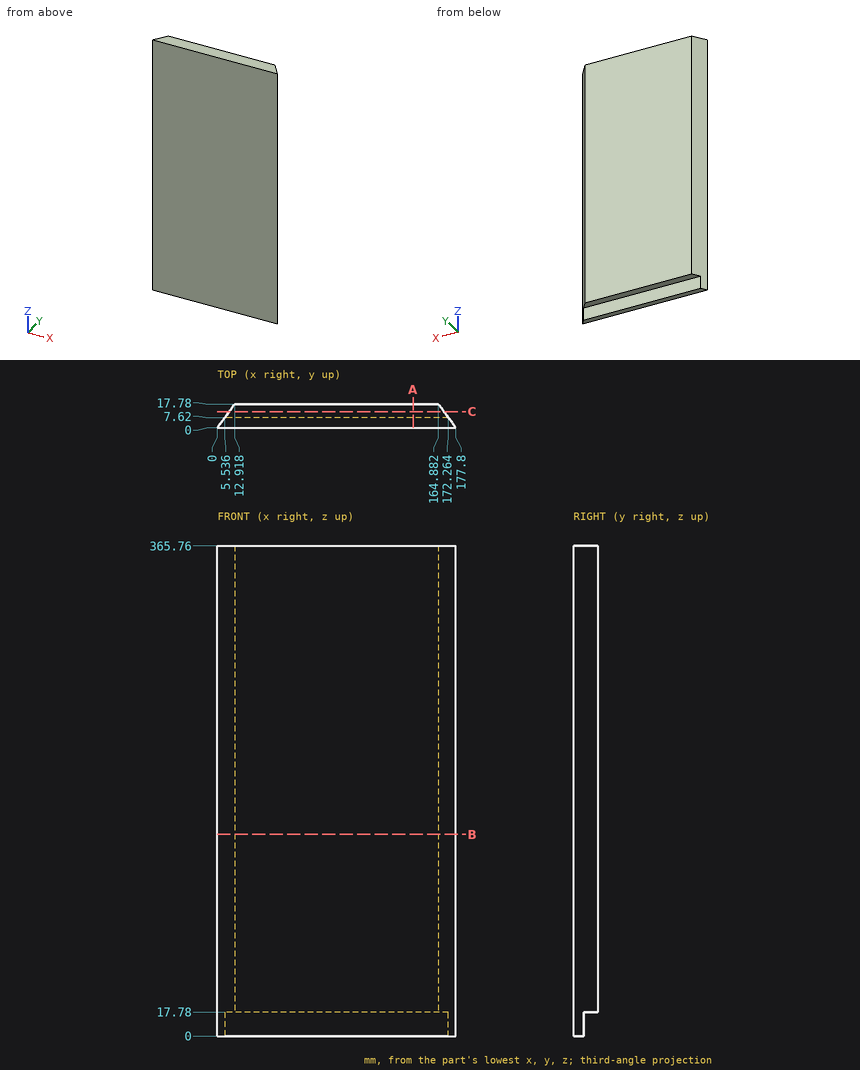
Geometry check sheet. Reference: drawing and pictorial views, mm from the part's lowest x, y, z. Give positions to 0.01 mm unless a question says otherwise; leave off trailing zeros. Loops run counter-clockwise (first coordinate to the right, second up) from the corner with the lowest first, then second, coordinate; pieces in that order, holes last. Notation, with made-up numbers: M 33.25,70.5 L 72.25,70.5 A18 cw 72.25,81.5 Z; hole C 57,70.5 d9. An arc over 180 degrees is marked long. One line per question, with ' | ' between items.
Item 1: Section check A-A, the plane x = 146. Record the cut outline in (y, z).
Completed:
outline: M 0,0 L 7.62,0 L 7.62,17.78 L 17.78,17.78 L 17.78,365.76 L 0,365.76 Z
Item 2: Section check C-C, the plane y = 12. Record the cut outline in (x, z).
Completed:
outline: M 8.72,17.78 L 169.08,17.78 L 169.08,365.76 L 8.72,365.76 Z
Item 3: Thickness scan on line 1 (Z direction, x = 160.5, y = 10); line 2 (X direction, y = 11.25, z = 64.5); line 3 (X direction, y = 7.75, z = 206). Record the ranges inside material, lowest first. Write a range as [from, to].
Completed:
line 1: z = [17.78, 365.76] | line 2: x = [8.17, 169.63] | line 3: x = [5.63, 172.17]
Item 4: Depth check by flat-ended pin: P1, Ø1.5, axis at y = 5.5, z = 237.5, coming from the -X side; P2, Ø2, axis at y = 5, z = 135, coming from the +X side; P3, Ø5, axis at x = 123, y = 12.5, coming from the -Z side. Enter the tip coordinate at first touch or a pass-through.
Completed:
P1: stops at x = 3.45 | P2: stops at x = 174.89 | P3: stops at z = 17.78
Item 5: Section check B-B, the plane z = 150.5. Record the cut outline in (x, y), plus the area to 3 significant figures.
Completed:
outline: M 0,0 L 177.8,0 L 164.88,17.78 L 12.92,17.78 Z | area: 2,930 mm^2
